from build123d import *

# Parameters (mm, degrees)
SKETCH1_W           = 232
SKETCH1_H           = 75
SKETCH1_R           = 2
BOSS_EXTRUDE1_DEPTH = 3.175
SKETCH2_W           = 50
SKETCH2_H           = 3.175
BOSS_EXTRUDE2_DEPTH = 3.175


with BuildPart() as part:
    # Sketch1 → Boss-Extrude1 (new body)
    with BuildSketch(Plane.XY):
        with Locations((116, 37.5)):
            Rectangle(SKETCH1_W, SKETCH1_H)
        with Locations((9, 65)):
            Circle(SKETCH1_R, mode=Mode.SUBTRACT)
        with Locations(Location((9, 10, 0), (0, 0, 180))):
            Circle(SKETCH1_R, mode=Mode.SUBTRACT)
        with Locations((223, 10)):
            Circle(SKETCH1_R, mode=Mode.SUBTRACT)
        with Locations(Location((223, 65, 0), (0, 0, 180))):
            Circle(SKETCH1_R, mode=Mode.SUBTRACT)
    extrude(amount=BOSS_EXTRUDE1_DEPTH)

    # Sketch2 → Boss-Extrude2 (add)
    with BuildSketch(Plane.XY.offset(3.175)):
        with Locations((116, -1.5875)):
            Rectangle(SKETCH2_W, SKETCH2_H)
        with Locations((116, 76.5875)):
            Rectangle(SKETCH2_W, SKETCH2_H)
    extrude(amount=-BOSS_EXTRUDE2_DEPTH)


solid = part.part
For this review, take the finished solid that the model builds, in its own axes (mm). Round coordinates to 2 decimals unless told otherwise and drop trailing zeros. Order: outer loops, then holes, each group sorted by start corner. A loop starts at its lowest first (then second) coordinate and runs counter-clockwise, first axis right, second up. Notation, with made-up numbers: M 39,15 L 97,15 A11 ccw 97,28 Z; hole C 3.5,7 d9. An arc over 180 degrees is marked long. Write each question's results on one line, items separated by ' | '. Start each with the question number.
1. Draft analysis for pull direction Y (two halves, no side actions). For faces 1 (the face through (9, 67, 2)), 2 (the face through (221, 10, 2)), 3 (the face through (114, 38, 3.175)), state which applies: pulls with the +Y half, pulls with the -Y half, needs draft (parallel to the pull), parting line crosses it, or undercut.
2. Clearance check with flat-ended pins moving along their axes: pin 1 Ø1.6 at (x, z) = (44.5, 1) entering from +Y; pin 2 Ø1.6 at (y, z) = (76, 1.5) entering from +X; pin 3 Ø2.5 at (x, y) = (9, 65) entering from -Z; pin 4 Ø1 at (x, z) = (190.5, 1.5) entering from -Y. State where each tip first meets the part, or that it passes through.
3. Add section C-C (y = 65). State the section outline as (x, z) points (3 decimals).
4. To check wall thickness, follow L1, parallel to Y at x = 223, z = 0.7; L2, parallel to Y at x = 10.5, z = 1.8; L3, parallel to Y at x = 33, z = 0.75. State the ranges of each line that lie inside material, in increasing order. Write a range as [from, to].
5. Add section A-A (x = 9). State the section outline as (y, z) points (3 decimals), then the cut area to 3 significant figures.
6. Add section D-D (x = 169.5). State the section outline as (y, z) points (3 decimals), then the cut area to 3 significant figures.
7. Add section B-B (z = 1.2). State the section outline as (x, y) points (3 decimals), then the cut area to 3 significant figures.
Output values:
1) face 1: undercut | face 2: undercut | face 3: needs draft
2) pin 1: y = 75 | pin 2: x = 141 | pin 3: through | pin 4: y = 0
3) outline: M 0,0 L 7,0 L 7,3.175 L 0,3.175 Z; M 11,0 L 221,0 L 221,3.175 L 11,3.175 Z; M 225,0 L 232,0 L 232,3.175 L 225,3.175 Z
4) L1: [0, 8], [12, 63], [67, 75] | L2: [0, 8.68], [11.32, 63.68], [66.32, 75] | L3: [0, 75]
5) outline: M 0,0 L 8,0 L 8,3.175 L 0,3.175 Z; M 12,0 L 63,0 L 63,3.175 L 12,3.175 Z; M 67,0 L 75,0 L 75,3.175 L 67,3.175 Z | area: 213 mm^2
6) outline: M 0,0 L 75,0 L 75,3.175 L 0,3.175 Z | area: 238 mm^2
7) outline: M 0,0 L 91,0 L 91,-3.175 L 141,-3.175 L 141,0 L 232,0 L 232,75 L 141,75 L 141,78.175 L 91,78.175 L 91,75 L 0,75 Z; hole C 9,10 d4; hole C 9,65 d4; hole C 223,10 d4; hole C 223,65 d4 | area: 17,700 mm^2
